```python
from build123d import *

# Parameters (mm, degrees)
SALIENTE_EXTRUIR1_DEPTH = 10
CROQUIS2_R              = 5
SALIENTE_EXTRUIR2_DEPTH = 20
REDONDEO1_R             = 2


with BuildPart() as part:
    # Croquis1 → Saliente-Extruir1 (new body)
    with BuildSketch(Plane.XY):
        with BuildLine():
            Line((-5.5, 37.599867021), (-5.5, 15.577785413))
            ThreePointArc((-5.5, 15.577785413), (0, 10.077785413), (5.5, 15.577785413))
            Line((5.5, 15.577785413), (5.5, 37.599867021))
            ThreePointArc((5.5, 37.599867021), (8.313819384, 37.079379812), (11.080493617, 36.348626676))
            ThreePointArc((11.080493617, 36.348626676), (18.9363196, 18.9363196), (36.348626676, 11.080493617))
            ThreePointArc((36.348626676, 11.080493617), (37.079379812, 8.313819384), (37.599867021, 5.5))
            Line((37.599867021, 5.5), (15.577785413, 5.5))
            ThreePointArc((15.577785413, 5.5), (10.077785413, 0), (15.577785413, -5.5))
            Line((15.577785413, -5.5), (37.599867021, -5.5))
            ThreePointArc((37.599867021, -5.5), (37.079379812, -8.313819384), (36.348626676, -11.080493617))
            ThreePointArc((36.348626676, -11.080493617), (18.9363196, -18.9363196), (11.080493617, -36.348626676))
            ThreePointArc((11.080493617, -36.348626676), (8.313819384, -37.079379812), (5.5, -37.599867021))
            Line((5.5, -37.599867021), (5.5, -15.577785413))
            ThreePointArc((5.5, -15.577785413), (0, -10.077785413), (-5.5, -15.577785413))
            Line((-5.5, -15.577785413), (-5.5, -37.599867021))
            ThreePointArc((-5.5, -37.599867021), (-8.313819384, -37.079379812), (-11.080493617, -36.348626676))
            ThreePointArc((-11.080493617, -36.348626676), (-18.9363196, -18.9363196), (-36.348626676, -11.080493617))
            ThreePointArc((-36.348626676, -11.080493617), (-37.079379812, -8.313819384), (-37.599867021, -5.5))
            Line((-37.599867021, -5.5), (-15.577785413, -5.5))
            ThreePointArc((-15.577785413, -5.5), (-10.077785413, 0), (-15.577785413, 5.5))
            Line((-15.577785413, 5.5), (-37.599867021, 5.5))
            ThreePointArc((-37.599867021, 5.5), (-37.079379812, 8.313819384), (-36.348626676, 11.080493617))
            ThreePointArc((-36.348626676, 11.080493617), (-18.9363196, 18.9363196), (-11.080493617, 36.348626676))
            ThreePointArc((-11.080493617, 36.348626676), (-8.313819384, 37.079379812), (-5.5, 37.599867021))
        make_face()
    extrude(amount=SALIENTE_EXTRUIR1_DEPTH)

    # Croquis2 → Saliente-Extruir2 (add)
    with BuildSketch(Plane(origin=(0, 0, 0), x_dir=(-1, 0, 0), z_dir=(0, 0, -1))):
        with Locations(Location((0, 0, 0), (0, 0, 180))):
            Circle(CROQUIS2_R)
    extrude(amount=SALIENTE_EXTRUIR2_DEPTH)

    # Redondeo1
    redondeo1_edges = [part.edges().sort_by_distance(p)[0] for p in [
        (-5.5, -37.599867021, 5),
        (-37.599867021, -5.5, 5),
        (-37.599867021, 5.5, 5),
        (-5.5, 37.599867021, 5),
        (5.5, 37.599867021, 5),
        (37.599867021, 5.5, 5),
        (37.599867021, -5.5, 5),
        (5.5, -37.599867021, 5),
    ]]
    fillet(redondeo1_edges, radius=REDONDEO1_R)


solid = part.part
```
Read the model definition and answer for the solid it produces. Units are mm, in the model's axes. A direction names the side the tool comes from. Coordinates: 2 decimals unless noted, no trailing zeros. Write each loop counter-clockwise with the first axis right and the second up, starting at its lowest first coordinate (ties: lowest second). Pieces come first, ordered by that corner, then holes. Notation, with made-up numbers: (-31, -16) -> (8, -16) arc R25 cw to (8, 18) -> close; hole circle Ø8 at (5, 27.5). An arc over 180 degrees is marked (long way). Return JSON: item names as keys, results as strings.
1. Find the intervals of material crossed by line 1 along Z through (x, y) = (4.5, 10.5); line 2 along Y through (x, z) = (7, 6); line 3 along X through (y, z) = (-24, 5.5), in increasing order. Write a range as from..to.
Found:
{"line 1": "0..10", "line 2": "-37.15..37.15", "line 3": "-14.96..-5.5, 5.5..14.96"}
2. A cutting plane is placed at C-C (y = 0). Determine the outline of the cut face in (x, z).
Found:
{"outline": "(-10.08, 0) -> (-5, 0) -> (-5, -20) -> (5, -20) -> (5, 0) -> (10.08, 0) -> (10.08, 10) -> (-10.08, 10) -> close"}
3. A tool of negligible diameter and unlimited length cuts with its end or side. For faces 1 (the face through (-25, 5.5, 5)), 2 (the face through (5.5, -26, 5)), 3 (the face through (36.749, -6.222, 5.07)), 4 (the face through (19.131, -18.744, 4.93)), 5 (the face through (-5.5, 26, 5)), from which of +Z, -Z, +X, -X, +Y, -Y can it reach the whole face along a straight path? Write none if from no direction.
Found:
{"face 1": "+Z, -Z, -X", "face 2": "+Z, -Z, -Y", "face 3": "+Z, -Z, +X", "face 4": "+Z, -Z, +X, -Y", "face 5": "+Z, -Z, +Y"}
4. Each of these flat-tipped pins is pushed along its axis until it touches: P1, Ø3, axis at x = 30, z = 3, coming from the -Y side; P2, Ø1.5, axis at y = 5, z = 1, coming from the +X side; P3, Ø8, axis at x = -21, z = 4.5, coming from the +Y side; P4, Ø1, axis at x = 3.5, y = 22, coming from the +Z side. Where does it stop, or does it pass through?
Found:
{"P1": "y = -12.77", "P2": "x = 36.18", "P3": "y = 21.09", "P4": "through"}
5. A cutting plane is placed at B-B (x = 31.5). Determine the outline of the cut face in (y, z).
Found:
{"outline": "(-11.83, 0) -> (-5.5, 0) -> (-5.5, 10) -> (-11.83, 10) -> close; (5.5, 0) -> (11.83, 0) -> (11.83, 10) -> (5.5, 10) -> close"}
6. Determine the mould class of faces 6 (the face through (26, 5.5, 5)), 7 (the face through (-5, 0, -10)), 8 (the face through (0.12, -10.08, 4.93)), 9 (the face through (-9.53, 36.786, 4.93)) for opening direction X: pulls with the +X half, pulls with the -X half, needs draft (parallel to the pull), parting line crosses it, or undercut.
Found:
{"face 6": "needs draft", "face 7": "parting line crosses it", "face 8": "undercut", "face 9": "pulls with the -X half"}
7. A cutting plane is placed at A-A (y = -14). Determine the outline of the cut face in (x, z).
Found:
{"outline": "(-25.71, 0) -> (-5.27, 0) -> (-5.27, 10) -> (-25.71, 10) -> close; (5.27, 0) -> (25.71, 0) -> (25.71, 10) -> (5.27, 10) -> close"}
